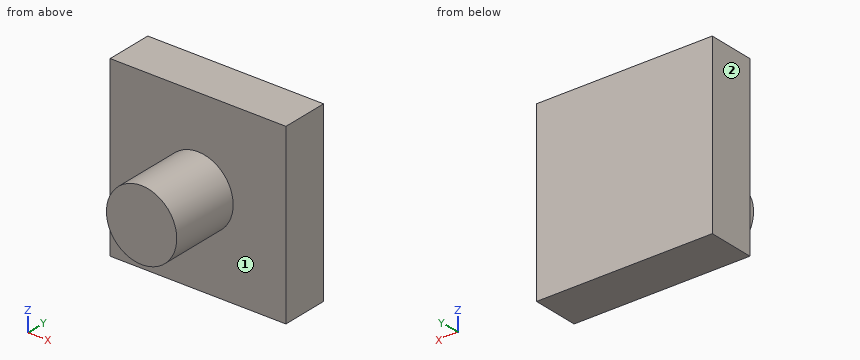
```python
from build123d import *

# Parameters (mm, degrees)
SKETCH1_W           = 30
SKETCH1_H           = 30
BOSS_EXTRUDE1_DEPTH = 8
SKETCH2_R           = 6
BOSS_EXTRUDE2_DEPTH = 12


with BuildPart() as part:
    # Sketch1 → Boss-Extrude1 (new body)
    with BuildSketch(Plane(origin=(0, 0, 0), x_dir=(1, 0, 0), z_dir=(0, 1, 0))):
        Rectangle(SKETCH1_W, SKETCH1_H)
    extrude(amount=BOSS_EXTRUDE1_DEPTH)

    # Sketch2 → Boss-Extrude2 (add)
    with BuildSketch(Plane(origin=(0, 0, 0), x_dir=(1, 0, 0), z_dir=(0, 1, 0))):
        with Locations(Location((0, 0, 0), (0, 0, 270))):
            Circle(SKETCH2_R)
    extrude(amount=-BOSS_EXTRUDE2_DEPTH)


solid = part.part
```
Source: CAD feature listing. Evaluate the final solid. Frame: model axes, mm. Face numbers are marked on the shaded views. A direction names the side the tool comes from. Give positions to 0.01 mm unless a question says otherwise; leave off trailing zeros. Loops run counter-clockwise (first coordinate to the right, second up) from the corner with the lowest first, then second, coordinate; pieces in that order, holes last. Notation, with made-up numbers: (11, -14.75) -> (65, -14.75) arc R9 ccw to (65, -3.75) -> close; hole circle Ø5 at (-26, -32). An arc over 180 degrees is marked (long way). Put each result on its own line as item: value. Start each with the question number.
1) Cut plane A-A (x = 0). Return loops of the section in (y, z).
2) Reachability of the marked faces 1 and 2 from +Z, -Z, +X, -X, +Y, -Y: full face, straight path, thin tool, end or side. Return the list, or none.
3) Contact query for flat-ended pins moving along their axis: P1, Ø4, axis at y = -1.5, z = 9, coming from the -X side; P2, Ø6, axis at x = -12, y = -3.5, coming from the -Z side; P3, Ø1, axis at x = 6, y = -5, coming from the -Z side; P4, Ø2, axis at x = -2.5, y = -4, coming from the -Z side. Output: stop coordinate, or through.
4) Cut plane B-B (z = 0). Return loops of the section in (x, y), then the cut area to 3 significant figures.
5) Cut plane D-D (z = 6.75). Return loops of the section in (x, y), then the cut area to 3 significant figures.
6) Cut plane C-C (y = -3.5). Return loops of the section in (x, z), then the cut area to 3 significant figures.
7) Material intervals for probe 1 along Y at (x, z) = (-6, -6); probe 2 along Z at (x, y) = (0.25, -2.25); probe 3 along X at (y, z) = (-6.75, -1.25), sorted ascending.
Results are:
1. outline: (-12, -6) -> (0, -6) -> (0, -15) -> (8, -15) -> (8, 15) -> (0, 15) -> (0, 6) -> (-12, 6) -> close
2. face 1: -Y
2. face 2: +Z, -Z, -X, +Y, -Y
3. P1: stops at x = -15
3. P2: passes through
3. P3: stops at z = -2.4
3. P4: stops at z = -5.81
4. outline: (-15, 0) -> (-6, 0) -> (-6, -12) -> (6, -12) -> (6, 0) -> (15, 0) -> (15, 8) -> (-15, 8) -> close
4. area: 384 mm2
5. outline: (-15, 0) -> (15, 0) -> (15, 8) -> (-15, 8) -> close
5. area: 240 mm2
6. outline: circle Ø12 at (0, 0)
6. area: 113 mm2
7. probe 1: y = 0 to 8
7. probe 2: z = -5.99 to 5.99
7. probe 3: x = -5.87 to 5.87
